Could you check a few things on this model? Use its own coordinates, in mm. A direction names the side the tool comes from. Coordinates: 2 decimals unless noted, no trailing zeros. Write each loop counter-clockwise with the first axis right and the second up, starting at its lowest first coordinate (ties: lowest second). Pieces come first, ordered by that corner, then holes. Notation, with made-up numbers: M 66.25,-8.5 L 89.25,-8.5 A18 ccw 89.25,14.5 Z; hole C 29,63.5 d10. An arc over 180 degrees is marked long. Write item = value, one per line.
Autodesk Inventor part; units mm, degrees
ref_plane "YZ Plane" through (0, 0, 0) normal (1, 0, 0) x (0, 1, 0)
ref_plane "XZ Plane" through (0, 0, 0) normal (0, 1, 0) x (-1, 0, 0)
ref_plane "XY Plane" through (0, 0, 0) normal (0, 0, 1) x (1, 0, 0)
sketch "Sketch1" plane through (0, 0, 0) normal (0, 1, 0) x (-1, 0, 0)
  circle A0 centre (0, 0) radius 19.05
  dimension "d0" = 38.1
extrude "Extrusion1" add sketch "Sketch1" along normal blind 12.7
sketch "Sketch2" plane through (0, 12.7, 0) normal (0, 1, 0) x (1, 0, 0)
  circle A0 centre (-17.2164, 0) radius 1.2279
  circle A1 centre (0, -17.2164) radius 1.2279
  circle A2 centre (17.2164, 0) radius 1.2279
  circle A3 centre (0, 17.2164) radius 1.2279
  circle A4 centre (0, 0) radius 14.5525
  dimension "d5" = 360
extrude "Extrusion2" add sketch "Sketch2" along normal blind 12.7 contours A4
extrude "Extrusion3" cut sketch "Sketch2" against normal up to next contours A0 | A1 | A2 | A3
properties part number "7.2 part 2"
Item 1: Imagine slicing it at B-B (z = 0). Write out the boundary of the cut face in (x, y).
Numbers:
outline = M -19.05,0 L -18.44,0 L -18.44,12.7 L -19.05,12.7 Z; M -15.99,0 L 15.99,0 L 15.99,12.7 L 14.55,12.7 L 14.55,25.4 L -14.55,25.4 L -14.55,12.7 L -15.99,12.7 Z; M 18.44,0 L 19.05,0 L 19.05,12.7 L 18.44,12.7 Z
Item 2: If I drill on line 1 along Z through (x, y) = (0, 5.25); line 2 along Y through (x, z) = (15.5, 1.5); line 3 along X through (y, z) = (9.5, -4.5), over which ranges is the centre line in solid material (lowest first)?
Numbers:
line_1 = -19.05 to -18.44, -15.99 to 15.99, 18.44 to 19.05
line_2 = 0 to 12.7
line_3 = -18.51 to 18.51
Item 3: For faces 5 (the face through (-0.266, 6.439, 18.415)), 6 (the face through (-3.155, 18.961, -14.206)), which set-ups out of +Z, -Z, +X, -X, +Y, -Y let a thin tool reach every point of the face, with its end or its side?
Numbers:
face_5 = +Y, -Y
face_6 = +Y
Item 4: Imagine slicing it at C-C (y = 13.75). Write out the boundary of the cut face in (x, z) (1 decimal).
Numbers:
outline = C 0,0 d29.1
Item 5: Imagine slicing it at D-D (z = -6.5). Write out the boundary of the cut face in (x, y), and give its area (3 significant figures).
Numbers:
outline = M -17.91,0 L 17.91,0 L 17.91,12.7 L 13.02,12.7 L 13.02,25.4 L -13.02,25.4 L -13.02,12.7 L -17.91,12.7 Z
area = 786 mm²
Item 6: I'm going to push flat-ended pins straight in: P1, Ø1, axis at y = 15, z = 4.5, coming from the +X side; P2, Ø5, axis at x = -6.5, y = 12, coming from the +Z side; P3, Ø1, axis at x = -7.5, y = 5, coming from the -Z side; P4, Ø2, axis at x = 17.22, z = 0, coming from the +Y side. Where does each tip first touch, or does it pass through?
Numbers:
P1 = 13.99
P2 = 18.63
P3 = -17.72
P4 = through
Item 7: Imagine slicing it at A-A (x = 0). Write out the boundary of the cut face in (y, z), and give its area (3 significant figures).
Numbers:
outline = M 0,-19.05 L 12.7,-19.05 L 12.7,-18.44 L 0,-18.44 Z; M 0,-15.99 L 12.7,-15.99 L 12.7,-14.55 L 25.4,-14.55 L 25.4,14.55 L 12.7,14.55 L 12.7,15.99 L 0,15.99 Z; M 0,18.44 L 12.7,18.44 L 12.7,19.05 L 0,19.05 Z
area = 791 mm²
Item 8: If we mould it in two halves opening along Z, with no side actions, what happens to faces 1 (the face through (15.99, 6.44, -0.05)), 2 (the face through (15.12, 6.26, 11.59)), 3 (the face through (0, 25.4, 0)), 4 (the face through (-0.27, 6.44, -16.02))? For each: pulls with the +Z half, pulls with the -Z half, needs draft (parallel to the pull), parting line crosses it, or undercut.
Numbers:
face_1 = undercut
face_2 = parting line crosses it
face_3 = needs draft
face_4 = undercut
